The model under review builds one solid part; all positions refer to its coordinate system, in mm. Coordinates: 2 decimals unless noted, no trailing zeros. Write each loop counter-clockwise with the first axis right and the second up, starting at its lowest first coordinate (ties: lowest second). Pieces come first, ordered by that corner, then holes. Notation, with made-up numbers: (8.25, 56) -> (58.25, 56) arc R24 ccw to (58.25, 72) -> close; hole circle Ø11 at (46.25, 19). An arc over 180 degrees is marked (long way). Put each result on its own line as item: value. Start each with the question number.
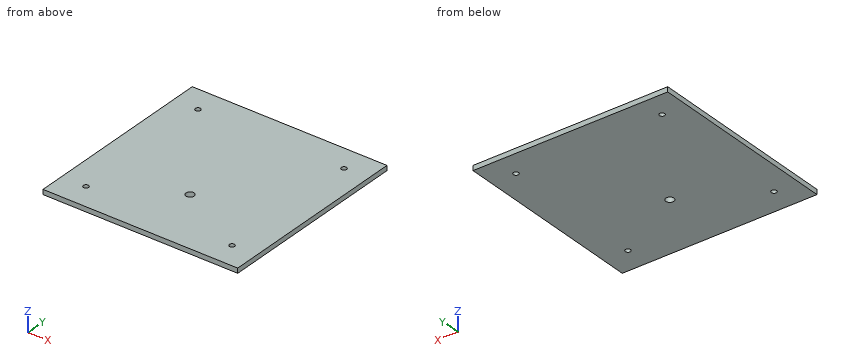
Solid Edge part; units mm, degrees
sketch "Sketch1" plane through (0, 0, 0) normal (0, 0, 1) x (1, 0, 0)
  line L0 (60, -60) -> (-60, -60)
  line L1 (-60, -60) -> (-60, 60)
  line L2 (-60, 60) -> (60, 60)
  line L3 (60, 60) -> (60, -60)
  dimension "D1" = 60
  dimension "D2" = 60
extrude "Protrusion1" add sketch "Sketch1" along normal blind 3
hole "Hole_1" at (0, -20, 3) direction (0, 0, -1) diameter 5 end through all
hole "Hole_2" at (-45, -45, 3) direction (0, 0, -1) diameter 3.2 end through all
hole "Hole1" at (45, -45, 3) direction (0, 0, -1) diameter 3.2 end through all
hole "Hole2" at (45, 45, 3) direction (0, 0, -1) diameter 3.2 end through all
hole "Hole3" at (-45, 45, 3) direction (0, 0, -1) diameter 3.2 end through all
1. Consider section A-A on x = 0. State the section outline as (y, z) points.
2. Insertion check: P1, Ø6, axis at x = 0, y = -20, coming from the -Z side; P2, Ø1.9, axis at x = -45, y = -45, coming from the +Z side. Each pin has a flat end and moves straight along its axis. Give the tip position at first contact, or say it passes through.
3. Consider section B-B on y = 45. State the section outline as (x, z) points.
4. Consider section D-D on y = -20. State the section outline as (x, z) points, then the cut area to 3 significant figures.
5. Wall thickness on line 1 (X direction, y = -45, z = 2.3); line 2 (X direction, y = -20, z = 1.05): over which ranges is each line inside the solid? List them lowest first. Write a range as from..to.
Output values:
1. outline: (-60, 0) -> (-22.5, 0) -> (-22.5, 3) -> (-60, 3) -> close; (-17.5, 0) -> (60, 0) -> (60, 3) -> (-17.5, 3) -> close
2. P1: stops at z = 0
2. P2: passes through
3. outline: (-60, 0) -> (-46.6, 0) -> (-46.6, 3) -> (-60, 3) -> close; (-43.4, 0) -> (43.4, 0) -> (43.4, 3) -> (-43.4, 3) -> close; (46.6, 0) -> (60, 0) -> (60, 3) -> (46.6, 3) -> close
4. outline: (-60, 0) -> (-2.5, 0) -> (-2.5, 3) -> (-60, 3) -> close; (2.5, 0) -> (60, 0) -> (60, 3) -> (2.5, 3) -> close
4. area: 345 mm^2
5. line 1: x = -60..-46.6, -43.4..43.4, 46.6..60
5. line 2: x = -60..-2.5, 2.5..60
